Part model, mm, in its own coordinate system. Face numbers are marked on the shaded views. A direction names the side the tool comes from. Give positions to 0.01 mm unless a question says otherwise; leave off trailing zeros. Order: outer loops, then holes, each group sorted by start corner. A loop starts at its lowest first (then second) coordinate and runs counter-clockwise, first axis right, second up. Notation, with made-up numbers: (50, 15) - (104, 15) arc R16 ccw to (104, 29) - close; hole circle Ø5 at (67, -27.5). An arc over 180 degrees is marked (long way). Use a Markdown table: item, result. Add a question column.
from build123d import *

# Parameters (mm, degrees)
F1_W     = 640.876718
F1_H     = 370.186116
F2_DEPTH = 330
F0_W     = 295.364954
F0_H     = 178.202663
F3_DEPTH = 345


with BuildPart() as f2:
    # F1 (on Top) → F2 (new body)
    with BuildSketch(Plane.XY):
        with Locations((242.221858, -144.041853)):
            Rectangle(F1_W, F1_H)
    extrude(amount=F2_DEPTH)

    # F0 (on Top) → F3 (join)
    with BuildSketch(Plane.XY):
        with Locations((51.913496, -36.990968)):
            Rectangle(F0_W, F0_H)
    extrude(amount=F3_DEPTH)


solid = f2.part
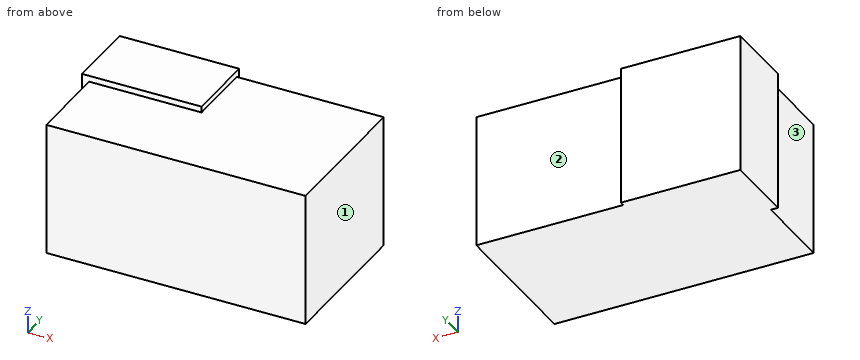
1. Cut at D-D (x = 429.5). Write the cut outline in (y, z), plus the area to 3 significant figures.
2. Drill centre lines: probe 1 along Z at (x, y) = (302, -183); probe 2 along X at (y, z) = (-174.5, 129.5); probe 3 along Y at (x, z) = (341, 197). Where is each one in solid material? Low to high. Write a range as [from, to].
3. Tool access for the marked faces 1, 2 and 3: list every direction of +Z, -Z, +X, -X, +Y, -Y with a clear straight run to the whole face (end or side of a thin tool).
4. Cut at C-C (y = 18). Write the cut outline in (x, z).
5. Cut at B-B (x = 171.5). Write the cut outline in (y, z).
6. Cut at A-A (z = 57). Write the cut outline in (x, y), plus the area to 3 significant figures.
7. Pin check, flat tips, straight feed: P1, Ø8, axis at x = 328.5, z = 294.5, coming from the +Y side; P2, Ø4, axis at y = -208, z = 254.5, coming from the -X side. Stop position of each tip, or through.
Responses:
| question | item | result |
|---|---|---|
| 1 | outline | (-329.13, 0) - (41.05, 0) - (41.05, 330) - (-329.13, 330) - close |
| 1 | area | 122,000 mm² |
| 2 | probe 1 | z = [0, 330] |
| 2 | probe 2 | x = [-78.22, 562.66] |
| 2 | probe 3 | y = [-329.13, 41.05] |
| 3 | face 1 | +Z, -Z, +X, +Y, -Y |
| 3 | face 2 | +Z, -Z, +X, +Y |
| 3 | face 3 | +Z, -Z, -X, -Y |
| 4 | outline | (-95.77, 0) - (562.66, 0) - (562.66, 330) - (199.6, 330) - (199.6, 345) - (-95.77, 345) - close |
| 5 | outline | (-329.13, 0) - (52.11, 0) - (52.11, 345) - (-126.09, 345) - (-126.09, 330) - (-329.13, 330) - close |
| 6 | outline | (-95.77, -126.09) - (-78.22, -126.09) - (-78.22, -329.13) - (562.66, -329.13) - (562.66, 41.05) - (199.6, 41.05) - (199.6, 52.11) - (-95.77, 52.11) - close |
| 6 | area | 243,000 mm² |
| 7 | P1 | stops at y = 41.05 |
| 7 | P2 | stops at x = -78.22 |
